from build123d import *

# Parameters (mm, degrees)
SKETCH_1_R      = 1.65
SKETCH_1_R_2    = 2.65
EXTRUDE_1_DEPTH = 3
FILLET_1_R      = 2.5


with BuildPart() as part:
    # 草图1 → 凸台-拉伸1 (new body)
    with BuildSketch(Plane(origin=(0, 0, 0), x_dir=(1, 0, 0), z_dir=(0, 1, 0))):
        Polygon((0, 0), (143, 0), (143, 37), (75, 37), (75, 30), (0, 30), align=None)
        with Locations(Location((10, 25, 0), (0, 0, 270))):
            Circle(SKETCH_1_R, mode=Mode.SUBTRACT)
        with Locations(Location((10, 6.37, 0), (0, 0, 270))):
            Circle(SKETCH_1_R, mode=Mode.SUBTRACT)
        with Locations(Location((50, 15, 0), (0, 0, 270))):
            Circle(SKETCH_1_R_2, mode=Mode.SUBTRACT)
        with Locations(Location((25, 15, 0), (0, 0, 270))):
            Circle(SKETCH_1_R, mode=Mode.SUBTRACT)
        with Locations(Location((100, 29.5, 0), (0, 0, 270))):
            Circle(SKETCH_1_R_2, mode=Mode.SUBTRACT)
        with Locations(Location((85.6, 8, 0), (0, 0, 270))):
            Circle(SKETCH_1_R, mode=Mode.SUBTRACT)
        with Locations(Location((133, 25, 0), (0, 0, 270))):
            Circle(SKETCH_1_R, mode=Mode.SUBTRACT)
        with Locations(Location((133, 6.37, 0), (0, 0, 270))):
            Circle(SKETCH_1_R, mode=Mode.SUBTRACT)
    extrude(amount=EXTRUDE_1_DEPTH)

    # 圆角1
    fillet_1_edges = [part.edges().sort_by_distance(p)[0] for p in [
        (0, 1.5, -30),
        (75, 1.5, -30),
        (75, 1.5, -37),
        (143, 1.5, -37),
        (143, 1.5, 0),
        (0, 1.5, 0),
    ]]
    fillet(fillet_1_edges, radius=FILLET_1_R)


solid = part.part
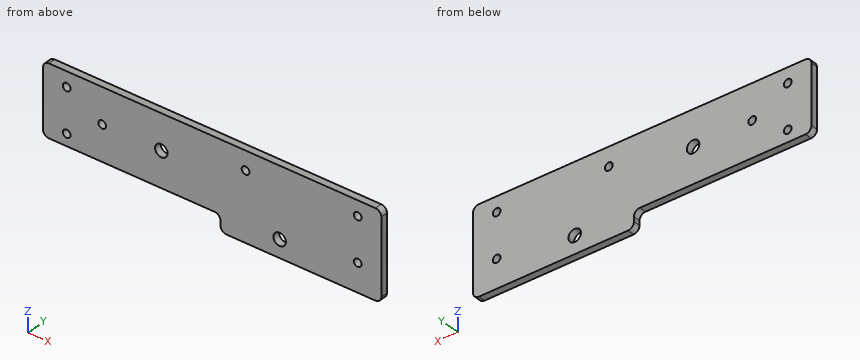
Model file for the job. Use its own axes, mm. Round coordinates to 2 decimals unless told otherwise and drop trailing zeros. Order: outer loops, then holes, each group sorted by start corner. A loop starts at its lowest first (then second) coordinate and runs counter-clockwise, first axis right, second up. Notation, with made-up numbers: M -30.5,82.5 L 14.5,82.5 A19 ccw 14.5,97.5 Z; hole C 1.5,14.5 d11. An arc over 180 degrees is marked long. Write each question's results on one line, items separated by ' | '. Start each with the question number.
(1) Saw through at B-B, the plane z = -15. Give the cut face in (x, y), then the cut area to 3 significant figures.
(2) Saw through at D-D, the plane y = 0.45. State how many separate pieces and enclosed holes the cut face has, then the cut area to 3 significant figures.
(3) Saw through at C-C, the plane x = 85.6. Give the cut face in (y, z).
(4) Probe probe 1 along Z at (x, y) = (133, 1.1); probe 2 along X at (y, z) = (1.25, -25); probe 3 along X at (y, z) = (1.85, -7.5). List the from-to ranges inside material, lowest first. Write a range as from..to.
(5) Drop flat-ended pins along their axis: pin 1 (7 mm diameter, centred on x = 100, z = -29.5, fed in from -Y); pin 2 (0.9 mm diameter, centred on x = 50, y = 1.5, fed in from -Z); pin 3 (2.5 mm diameter, centred on x = 133, z = -6.37, fed in from +Y) (3 decimals); pin 4 (1 mm diameter, centred on y = 2, z = -33.5, fed in from -X). Give the stop position or say it passes through.
(6) Saw through at A-A, the plane x = 10. Give the cut face in (y, z).
Established:
1) outline: M 0,0 L 23.35,0 L 23.35,3 L 0,3 Z; M 26.65,0 L 47.35,0 L 47.35,3 L 26.65,3 Z; M 52.65,0 L 143,0 L 143,3 L 52.65,3 Z | area: 403 mm^2
2) separate pieces: 1 | enclosed holes: 8 | area: 4,670 mm^2
3) outline: M 0,-37 L 3,-37 L 3,-9.65 L 0,-9.65 Z; M 0,-6.35 L 3,-6.35 L 3,0 L 0,0 Z
4) probe 1: z = -37..-26.65, -23.35..-8.02, -4.72..0 | probe 2: x = 0..8.35, 11.65..131.35, 134.65..143 | probe 3: x = 0..8.8, 11.2..84.03, 87.17..131.8, 134.2..143
5) pin 1: stops at y = 0 | pin 2: stops at z = -30 | pin 3: passes through | pin 4: stops at x = 75
6) outline: M 0,-30 L 3,-30 L 3,-26.65 L 0,-26.65 Z; M 0,-23.35 L 3,-23.35 L 3,-8.02 L 0,-8.02 Z; M 0,-4.72 L 3,-4.72 L 3,0 L 0,0 Z
